For this review, take the finished solid that the model builds, in its own axes (mm). Give positions to 0.01 mm unless a question says otherwise; leave off trailing zeros. Loops run counter-clockwise (first coordinate to the right, second up) from the corner with the lowest first, then second, coordinate; pieces in that order, holes last. Notation, with made-up numbers: (86.25, -9) - (96.25, -9) arc R19 cw to (96.25, 22) - close; hole circle Ø9 at (59, 24). An arc over 180 degrees is marked (long way). Put each result on its own line as item: value. Start each with the question number.
from build123d import *

# Parameters (mm, degrees)
F0_R     = 29.25
F1_DEPTH = 0.5
F2_D     = 3


with BuildPart() as f1:
    # F0 (on Front) → F1 (new body)
    with BuildSketch(Plane.XZ):
        Circle(F0_R)
        with BuildLine():
            ThreePointArc((14.588064, -1.62686), (8.45, -6.35), (2.311936, -1.62686))
            ThreePointArc((2.311936, -1.62686), (2.364165, -1.367049), (2.601923, -1.25))
            Line((2.601923, -1.25), (5.341946, -1.25))
            ThreePointArc((5.341946, -1.25), (8.45, -3.35), (11.558054, -1.25))
            Line((11.558054, -1.25), (14.298077, -1.25))
            ThreePointArc((14.298077, -1.25), (14.535835, -1.367049), (14.588064, -1.62686))
        make_face(mode=Mode.SUBTRACT)
        with BuildLine():
            ThreePointArc((-19.888064, 1.62686), (-7.4, 0), (-19.888064, -1.62686))
            ThreePointArc((-19.888064, -1.62686), (-19.835835, -1.367049), (-19.598077, -1.25))
            Line((-19.598077, -1.25), (-16.858054, -1.25))
            ThreePointArc((-16.858054, -1.25), (-10.4, 0), (-16.858054, 1.25))
            Line((-16.858054, 1.25), (-19.598077, 1.25))
            ThreePointArc((-19.598077, 1.25), (-19.835835, 1.367049), (-19.888064, 1.62686))
        make_face(mode=Mode.SUBTRACT)
        with BuildLine():
            Line((5.341946, 1.25), (2.601923, 1.25))
            ThreePointArc((2.601923, 1.25), (2.364165, 1.367049), (2.311936, 1.62686))
            ThreePointArc((2.311936, 1.62686), (8.45, 6.35), (14.588064, 1.62686))
            ThreePointArc((14.588064, 1.62686), (14.535835, 1.367049), (14.298077, 1.25))
            Line((14.298077, 1.25), (11.558054, 1.25))
            ThreePointArc((11.558054, 1.25), (8.45, 3.35), (5.341946, 1.25))
        make_face(mode=Mode.SUBTRACT)
    extrude(amount=F1_DEPTH)

    # F2 (through all)
    with Locations(Plane(origin=(0, 0, 0), x_dir=(1, 0, 0), z_dir=(0, 1, 0))):
        with Locations((-18.101934, 18.101934), (18.101934, 18.101934), (18.101934, -18.101934), (-18.101934, -18.101934)):
            Hole(F2_D / 2)


solid = f1.part
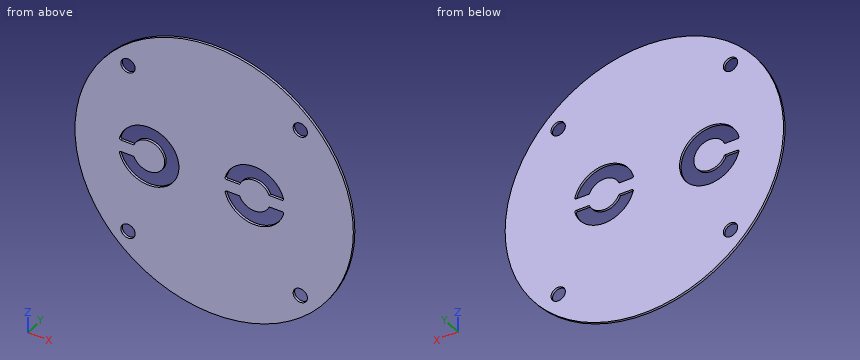
1) Take a section at A-A on z = 0. State the section outline as (x, y) points.
2) Take a section at B-B on x = 18. State the section outline as (y, z) points.
3) Insertion check: P1, Ø5, axis at x = -15, z = -21.5, coming from the +Y side. The pin has a flat end and moves straight along its axis. Give the tip position at first contact, or say it passes through.
4) Take a section at C-C on y = -0.25. State the section outline as (x, z) points.
5) Take a section at D-D on x = 4. State the section outline as (y, z) points, and give its area (3 significant figures).
6) Wall thickness on probe 1 along X at (y, z) = (-0.4, -1.5); probe 2 along X at (y, z) = (-0.1, -5.5); probe 3 along Z at (x, y) = (-17.5, -0.1): over which ranges is each line inside the solid? List them lowest first.
Answers follow:
1. outline: (-29.25, -0.5) - (-10.4, -0.5) - (-10.4, 0) - (-29.25, 0) - close; (-7.4, -0.5) - (29.25, -0.5) - (29.25, 0) - (-7.4, 0) - close
2. outline: (-0.5, -23.06) - (0, -23.06) - (0, -19.6) - (-0.5, -19.6) - close; (-0.5, -16.61) - (0, -16.61) - (0, 16.61) - (-0.5, 16.61) - close; (-0.5, 19.6) - (0, 19.6) - (0, 23.06) - (-0.5, 23.06) - close
3. P1: y = 0
4. outline: circle Ø58.5 at (0, 0); hole (-19.89, -1.63) arc R6.35 ccw (long way) to (-19.89, 1.63) arc R0.3 ccw to (-19.6, 1.25) - (-16.86, 1.25) arc R3.35 cw (long way) to (-16.86, -1.25) - (-19.6, -1.25) arc R0.3 ccw to start; hole circle Ø3 at (-18.1, -18.1); hole circle Ø3 at (-18.1, 18.1); hole (2.31, -1.63) arc R6.35 ccw to (14.59, -1.63) arc R0.3 ccw to (14.3, -1.25) - (11.56, -1.25) arc R3.35 cw to (5.34, -1.25) - (2.6, -1.25) arc R0.3 ccw to start; hole (2.31, 1.63) arc R0.3 ccw to (2.6, 1.25) - (5.34, 1.25) arc R3.35 cw to (11.56, 1.25) - (14.3, 1.25) arc R0.3 ccw to (14.59, 1.63) arc R6.35 ccw to start; hole circle Ø3 at (18.1, -18.1); hole circle Ø3 at (18.1, 18.1)
5. outline: (-0.5, -28.98) - (0, -28.98) - (0, -4.53) - (-0.5, -4.53) - close; (-0.5, -1.25) - (0, -1.25) - (0, 1.25) - (-0.5, 1.25) - close; (-0.5, 4.53) - (0, 4.53) - (0, 28.98) - (-0.5, 28.98) - close
5. area: 25.7 mm2
6. probe 1: -29.21 to -19.89, -16.75 to -10.75, -7.58 to 2.31, 5.45 to 11.45, 14.59 to 29.21
6. probe 2: -28.73 to -16.92, -10.58 to 5.28, 11.62 to 28.73
6. probe 3: -23.44 to -19.48, -16.73 to -5.12, -1.25 to 1.25, 5.12 to 16.73, 19.48 to 23.44
